from build123d import *

# Parameters (mm, degrees)
SKETCH1_R           = 16
SKETCH1_R_2         = 10
BOSS_EXTRUDE1_DEPTH = 7
FILLET1_R           = 0.5
SKETCH2_R           = 14.25
SKETCH2_R_2         = 11.75
CUT_EXTRUDE1_DEPTH  = 0.5
SKETCH3_R           = 14.25
SKETCH3_R_2         = 11.75
CUT_EXTRUDE2_DEPTH  = 0.5


with BuildPart() as part:
    # Sketch1 → Boss-Extrude1 (new body)
    with BuildSketch(Plane.XY):
        with Locations((80, 28.257283518)):
            Circle(SKETCH1_R)
        with Locations((80, 28.257283518)):
            Circle(SKETCH1_R_2, mode=Mode.SUBTRACT)
    extrude(amount=BOSS_EXTRUDE1_DEPTH)

    # Fillet1
    fillet1_edges = [part.edges().sort_by_distance(p)[0] for p in [
        (64, 28.257283518, 0),
        (64, 28.257283518, 7),
        (70, 28.257283518, 0),
        (70, 28.257283518, 7),
    ]]
    fillet(fillet1_edges, radius=FILLET1_R)

    # Sketch2 → Cut-Extrude1 (cut)
    with BuildSketch(Plane(origin=(0, 0, 0), x_dir=(-1, 0, 0), z_dir=(0, 0, -1))):
        with Locations((-80, 28.257283518)):
            Circle(SKETCH2_R)
        with Locations((-80, 28.257283518)):
            Circle(SKETCH2_R_2, mode=Mode.SUBTRACT)
    extrude(amount=-CUT_EXTRUDE1_DEPTH, mode=Mode.SUBTRACT)

    # Sketch3 → Cut-Extrude2 (cut)
    with BuildSketch(Plane.XY.offset(7)):
        with Locations((80, 28.257283518)):
            Circle(SKETCH3_R)
        with Locations((80, 28.257283518)):
            Circle(SKETCH3_R_2, mode=Mode.SUBTRACT)
    extrude(amount=-CUT_EXTRUDE2_DEPTH, mode=Mode.SUBTRACT)


solid = part.part
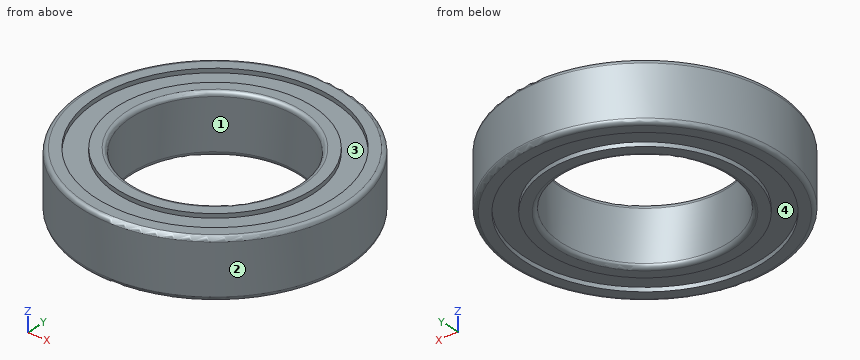
The listing builds one solid part. Answer for the finished solid, in the listing's coordinates (mm). Face numbers are marked on the shaded views. A direction names the side the tool comes from. Round coordinates to 2 decimals unless told otherwise and drop trailing zeros. Order: outer loops, then holes, each group sorted by start corner. A loop starts at its lowest first (then second) coordinate and runs counter-clockwise, first axis right, second up. Notation, with made-up numbers: (-36, 40) -> (15, 40) arc R23 ccw to (15, 64) -> close; hole circle Ø7 at (-31, 55.25). An arc over 180 degrees is marked (long way). Write each question's results on one line, items separated by ' | '. Start each with the question number.
Q1. The mould has two halves that part along X. Classify the marked faces 1 and 2: pulls with the +X half, pulls with the -X half, needs draft (parallel to the pull), parting line crosses it, or undercut.
Q2. Which of the six approach directions +Z, -Z, +X, -X, +Y, -Y give full straight-line access (tool end or side, diameter ignored) to the marked faces 3 and 4?
Q3. Each of these flat-tipped pins is pushed along its axis until it touches: pin 1 (4 mm diameter, centred on x = 84, z = 5.5, fed in from -Y); pin 2 (2 mm diameter, centred on x = 83.5, z = 2.5, fed in from +Y); pin 3 (4 mm diameter, centred on y = 17.5, z = 2.5, fed in from +X). Where does it stop, or does it pass through?
Q4. Straight lines are drawn through the part: probe 1 along X at (y, z) = (28, 1.5); probe 2 along Y at (x, z) = (77.5, 2.75); probe 3 along Y at (x, z) = (80, 3.3). For each, find the intervals that lie inside material, in ascending order. Write a range as from..to.
Q5. Find section B-B (z = 4.25). Determine the outline of the cut face in (x, y), then the cut area to 3 significant figures.
Worked answers:
1) face 1: undercut | face 2: parting line crosses it
2) face 3: +Z | face 4: -Z
3) pin 1: stops at y = 12.38 | pin 2: stops at y = 44.06 | pin 3: stops at x = 93.39
4) probe 1: x = 64..70, 90..96 | probe 2: y = 12.45..18.57, 37.94..44.06 | probe 3: y = 12.26..18.26, 38.26..44.26
5) outline: circle Ø32 at (80, 28.26); hole circle Ø20 at (80, 28.26) | area: 490 mm2
